Input: part model. Units: mm. Frame: model coordinates. A direction names the side the tool comes from. Coordinates: 2 decimals unless noted, no trailing zeros. Order: outer loops, then holes, each group sorted by start corner. A loop starts at its lowest first (then second) coordinate and runs counter-clockwise, first axis right, second up. Notation, with made-up numbers: M 37,2.25 L 85,2.25 A7 ccw 85,6.25 Z; hole C 53,56 d11. An arc over 180 degrees is marked long. One line per item, written item: value.
```python
from build123d import *

# Parameters (mm, degrees)
SKETCH1_W           = 19.05
SKETCH1_H           = 12.7
SKETCH1_W_2         = 9.525
SKETCH1_H_2         = 63.5
SKETCH1_W_3         = 3.175
SKETCH1_H_3         = 31.75
BOSS_EXTRUDE1_DEPTH = 31.75
CUT_EXTRUDE1_DEPTH  = 31.75
SKETCH3_R           = 4.7625
CUT_EXTRUDE2_DEPTH  = 31.75
SKETCH4_R           = 6.35
CUT_EXTRUDE3_DEPTH  = 100.595858348


with BuildPart() as part:
    # Sketch1 → Boss-Extrude1 (new body)
    with BuildSketch(Plane.XY):
        with Locations((-19.05, -57.15)):
            Rectangle(SKETCH1_W, SKETCH1_H)
        with Locations((-4.7625, -31.75)):
            Rectangle(SKETCH1_W_2, SKETCH1_H_2)
        with Locations((1.5875, -15.875)):
            Rectangle(SKETCH1_W_3, SKETCH1_H_3)
        Polygon((3.175, -31.75), (0, -31.75), (0, -44.45), (31.75, -44.45), (31.75, -31.75), (28.575, -31.75), align=None)
        with Locations((30.1625, -15.875)):
            Rectangle(SKETCH1_W_3, SKETCH1_H_3)
        Polygon((31.75, -31.75), (31.75, -44.45), (31.75, -63.5), (41.275, -63.5), (41.275, -50.8), (41.275, 0), (31.75, 0), align=None)
        with Locations((50.8, -57.15)):
            Rectangle(SKETCH1_W, SKETCH1_H)
    extrude(amount=BOSS_EXTRUDE1_DEPTH)

    # Sketch2 → Cut-Extrude1 (cut)
    with BuildSketch(Plane(origin=(0, -50.8, 0), x_dir=(1, 0, 0), z_dir=(0, 1, 0))):
        Polygon((-20.955, -31.75), (-28.575, -24.13), (-28.575, -31.75), align=None)
        Polygon((52.705, -31.75), (60.325, -24.13), (60.325, -31.75), align=None)
    extrude(amount=-CUT_EXTRUDE1_DEPTH, mode=Mode.SUBTRACT)

    # Sketch3 → Cut-Extrude2 (cut)
    with BuildSketch(Plane(origin=(0, -50.8, 0), x_dir=(1, 0, 0), z_dir=(0, 1, 0))):
        with Locations(Location((-19.05, -15.875, 0), (0, 0, 270))):
            Circle(SKETCH3_R)
        with Locations(Location((50.8, -15.875, 0), (0, 0, 270))):
            Circle(SKETCH3_R)
    extrude(amount=-CUT_EXTRUDE2_DEPTH, mode=Mode.SUBTRACT)

    # Sketch4 → Cut-Extrude3 (cut, through all)
    with BuildSketch(Plane(origin=(41.275, 0, 0), x_dir=(0, 0, -1), z_dir=(1, 0, 0))):
        with Locations((-15.875, -12.7)):
            Circle(SKETCH4_R)
        with BuildLine():
            Line((0, 0), (-15.875, 0))
            ThreePointArc((-15.875, 0), (-7.750642571, -0.876286908), (0, -3.464839036))
            Line((0, -3.464839036), (0, 0))
        make_face()
        with BuildLine():
            Line((-15.875, 0), (-31.75, 0))
            Line((-31.75, 0), (-31.75, -3.464839036))
            ThreePointArc((-31.75, -3.464839036), (-23.999357429, -0.876286908), (-15.875, 0))
        make_face()
    extrude(amount=-CUT_EXTRUDE3_DEPTH, mode=Mode.SUBTRACT)


solid = part.part
```
(1) Cut plane D-D on z = 17. Give the number of separate pieces and of enclosed holes in the cut face, plus the area to 3 significant figures.
Data:
separate pieces: 5
enclosed holes: 0
area: 1,750 mm2
(2) Draft query along Y for faces 1 (the cylindrical face through (35.01, -18.9, 17.25)), 2 (the flat face through (-9.525, -26, 16)), 3 (the flat face through (16, -31.75, 16)). Return one class per face: released by +Y, released by -Y, zero draft, split by the parting line, or undercut.
Data:
face 1: undercut
face 2: zero draft
face 3: released by +Y
(3) Access query for faces 4 (the flat face through (41.275, -26, 16)), 5 (the flat face through (3.175, -20, 16)), 6 (the flat face through (31.75, -54, 16)), 7 (the flat face through (-11, -63.5, 16)), 8 (the flat face through (-15, -50.8, 12)). Directions: +Z, -Z, +X, -X, +Y, -Y. A direction counts if a zero-diameter tool reaches every point of the face in a straight line with its end or side. Return the directions, or none.
Data:
face 4: +Z, -Z, +X, +Y
face 5: +Z, -Z, +Y
face 6: +Z, -Z, -Y
face 7: +Z, -Z, +X, -X, -Y
face 8: +Z, -Z, -X, +Y
(4) Cut plane A-A on y = -12.7. Output: boundary loops of the cut face in (x, z) (3 decimals).
Data:
outline: M -9.525,0 L 3.175,0 L 3.175,9.525 L -9.525,9.525 Z; M -9.525,22.225 L 3.175,22.225 L 3.175,31.75 L -9.525,31.75 Z; M 28.575,0 L 41.275,0 L 41.275,9.525 L 28.575,9.525 Z; M 28.575,22.225 L 41.275,22.225 L 41.275,31.75 L 28.575,31.75 Z
(5) Ray query, line 1 (X direction, y = -49.5, z = 11) (3 decimals); line 2 (X direction, y = -51, z = 2) (3 decimals); line 3 (Z direction, x = -19, y = -54). Return the intervals inside material, ascending. Write a range as from..to.
Data:
line 1: x = -9.525..0, 31.75..41.275
line 2: x = -28.575..0, 31.75..60.325
line 3: z = 0..11.11, 20.64..31.75
(6) Cut plane B-B on x = -19.05. Output: boundary loops of the cut face in (y, z).
Data:
outline: M -63.5,0 L -50.8,0 L -50.8,11.11 L -63.5,11.11 Z; M -63.5,20.64 L -50.8,20.64 L -50.8,31.75 L -63.5,31.75 Z
(7) First-contact query: pin 1 (2 mm diameter, centred on x = 17, z = 7.5, fed in from -Y); pin 2 (2 mm diameter, centred on x = 46.5, y = -55, fed in from -Z); pin 3 (1 mm diameter, centred on y = -43.5, z = 6.5, fed in from +X) (3 decimals); pin 4 (12.5 mm diameter, centred on x = 10, z = 18, fed in from +Y). Flat tips, straight axial feed; report the tip coordinate or a pass-through.
Data:
pin 1: stops at y = -44.45
pin 2: stops at z = 0
pin 3: stops at x = 41.275
pin 4: stops at y = -31.75
(8) Cut plane C-C on y = -21. Output: boundary loops of the cut face in (x, z) (3 decimals), plus the area to 3 significant figures.
Data:
outline: M -9.525,0 L 3.175,0 L 3.175,31.75 L -9.525,31.75 Z; M 28.575,0 L 41.275,0 L 41.275,31.75 L 28.575,31.75 Z
area: 806 mm2
